```python
from build123d import *

# Parameters (mm, degrees)
F0_W      = 44.45
F0_H      = 44.45
F1_DEPTH  = 76.2
F2_R      = 40.64
F4_R      = 12.7
F6_T      = -2.54
F3_W      = 17.78
F3_H      = 3.81
F7_DEPTH  = 5.08
F8_D      = 3.81
F8_DEPTH  = 5.08
F8_TIP    = 1.1446394792
F9_D      = 3.81
F9_DEPTH  = 5.08
F9_TIP    = 1.1446394792
F10_D     = 31.75
F10_DEPTH = 5.08
F10_TIP   = 9.5386623271


with BuildPart() as f1:
    # F0 (on Top) → F1 (new body)
    with BuildSketch(Plane.XY):
        with Locations((2.945480904, 3.0331164956)):
            Rectangle(F0_W, F0_H)
    extrude(amount=F1_DEPTH)

    # F2
    f2_edges = [f1.edges().sort_by_distance(p)[0] for p in [
        (2.945481, -19.191884, 76.2),
    ]]
    fillet(f2_edges, radius=F2_R)

    # F4
    f4_edges = [f1.edges().sort_by_distance(p)[0] for p in [
        (25.170481, -7.288703, 64.29682),
        (-19.279519, -7.288703, 64.29682),
    ]]
    fillet(f4_edges, radius=F4_R)

    # F6 (hollow: no face is removed)
    offset(amount=F6_T, mode=Mode.SUBTRACT)

    # F3 (on face) → F7 (cut)
    with BuildSketch(Plane(origin=(0, 25.2581164956, 0), x_dir=(-1, 0, 0), z_dir=(0, 1, 0))):
        with Locations((-2.945480904, 71.755)):
            Rectangle(F3_W, F3_H)
    extrude(amount=-F7_DEPTH, mode=Mode.SUBTRACT)

    # F8
    with Locations(Plane(origin=(0, 0, 0), x_dir=(1, 0, 0), z_dir=(0, 0, -1))):
        with Locations((18.820480904, 12.8418835044), (-12.929519096, 12.8418835044), (18.820480904, -18.9081164956), (-12.929519096, -18.9081164956)):
            Hole(F8_D / 2, depth=F8_DEPTH)
            with Locations((0, 0, -(F8_DEPTH + F8_TIP / 2))):  # 118° drill point
                Cone(0, F8_D / 2, F8_TIP, mode=Mode.SUBTRACT)

    # F9
    with Locations(Plane(origin=(0, 25.2581164956, 0), x_dir=(-1, 0, 0), z_dir=(0, 1, 0))):
        with Locations((-18.820480904, 40.64), (12.929519096, 40.64)):
            Hole(F9_D / 2, depth=F9_DEPTH)
            with Locations((0, 0, -(F9_DEPTH + F9_TIP / 2))):  # 118° drill point
                Cone(0, F9_D / 2, F9_TIP, mode=Mode.SUBTRACT)

    # F10
    with Locations(Plane(origin=(0, 0, 0), x_dir=(1, 0, 0), z_dir=(0, 0, -1))):
        with Locations((2.945480904, -3.0331164956)):
            Hole(F10_D / 2, depth=F10_DEPTH)
            with Locations((0, 0, -(F10_DEPTH + F10_TIP / 2))):  # 118° drill point
                Cone(0, F10_D / 2, F10_TIP, mode=Mode.SUBTRACT)


solid = f1.part
```
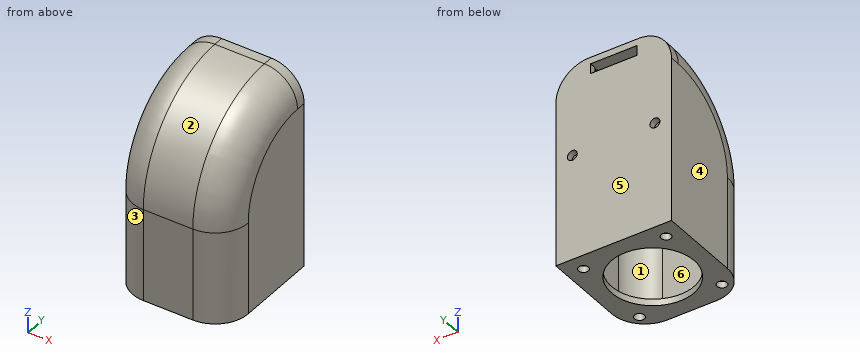
Geometry: final body of the model. Coordinates: model frame, mm. Face numbers are marked on the shaded views. A direction names the side the tool comes from. Coordinates: 2 decimals unless noted, no trailing zeros. Order: outer loops, then holes, each group sorted by start corner. A loop starts at its lowest first (then second) coordinate and runs counter-clockwise, first axis right, second up. Notation, with made-up numbers: (76.25, -39.75) -> (113.25, -39.75) arc R14 ccw to (113.25, -23.75) -> close; hole circle Ø4 at (60, 77). An arc over 180 degrees is marked (long way). Write item = value, one per line.
(1) Access query for the marked faces 1 and 2. Directions: +Z, -Z, +X, -X, +Y, -Y. A direction counts if a zero-diameter tool reaches every point of the face in a straight line with its end or side. Return the directions, or none.
Solved:
face_1 = none
face_2 = +Z, +X, -X, -Y
(2) Pin query (flat end, axial travel): pin 1 Ø19 at (x, y) = (2.95, 3.03) entering from +Z; pin 2 Ø2 at (y, z) = (24, 71) entering from -X; pin 3 Ø3 at (y, z) = (24.5, 72) entering from +X. Return the tip coordinate at first contact, or that it passes through.
Solved:
pin_1 = 75.21
pin_2 = -17.49
pin_3 = 23.07
(3) Cut plane A-A on z = 26. Return loops of the section in (x, y).
Solved:
outline = (-19.28, -6.49) arc R12.7 ccw to (-6.58, -19.19) -> (12.47, -19.19) arc R12.7 ccw to (25.17, -6.49) -> (25.17, 25.26) -> (-19.28, 25.26) -> close; hole (-16.74, -6.49) arc R10.16 ccw to (-6.58, -16.65) -> (12.47, -16.65) arc R10.16 ccw to (22.63, -6.49) -> (22.63, 22.72) -> (-16.74, 22.72) -> close
(4) Line query: line 1 (X direction, y = 12.5, z = 51); line 2 (X direction, y = 23, z = 40); line 3 (X direction, y = -9.5, z = 51). Output: solid intervals per line, ascending.
Solved:
line_1 = -19.28 to -16.74, 22.63 to 25.17
line_2 = -19.28 to -14.72, -11.14 to 17.03, 20.61 to 25.17
line_3 = -17.4 to -14.26, 20.16 to 23.29
(5) Pull-direction query (Y, two-part tool) for the marked faces 3, 4, 5 and 6; classes: pulls with the +Y half, pulls with the -Y half, needs draft (parallel to the pull), parting line crosses it, or undercut.
Solved:
face_3 = pulls with the -Y half
face_4 = needs draft
face_5 = pulls with the +Y half
face_6 = undercut
